```python
from build123d import *

# Parameters (mm, degrees)
F2_R = 12.599118
F3_R = 6.735102
F4_R = 3.026182
F5_R = 1.710135
F6_R = 1.408864


with BuildPart() as f1:
    # F0 (on Front) → F1 (revolve)
    with BuildSketch(Plane.XZ):
        Polygon((-9.7125, 0), (0, 0), (0, 22.078488), (-1.08705, 22.078488), (-3.406609, 20.364031), (-5.827018, 17.439371), (-6.936371, 12.598556), (-6.230419, 11.590051), (-7.944874, 11.18665), align=None)
    revolve(axis=Axis((0, 0, 11.039244), (0, 0, -1)))

    # F2
    f2_edges = [f1.edges().sort_by_distance(p)[0] for p in [
        (5.827018, 0, 17.439371),
    ]]
    fillet(f2_edges, radius=F2_R)

    # F3
    f3_edges = [f1.edges().sort_by_distance(p)[0] for p in [
        (3.406609, 0, 20.364031),
    ]]
    fillet(f3_edges, radius=F3_R)

    # F4
    f4_edges = [f1.edges().sort_by_distance(p)[0] for p in [
        (1.08705, 0, 22.078488),
    ]]
    fillet(f4_edges, radius=F4_R)

    # F5
    f5_edges = [f1.edges().sort_by_distance(p)[0] for p in [
        (7.944874, 0, 11.18665),
    ]]
    fillet(f5_edges, radius=F5_R)

    # F6
    f6_edges = [f1.edges().sort_by_distance(p)[0] for p in [
        (9.7125, 0, 0),
    ]]
    fillet(f6_edges, radius=F6_R)


solid = f1.part
```
For this review, take the finished solid that the model builds, in its own axes (mm). Round coordinates to 2 decimals unless told otherwise and drop trailing zeros. Loops run counter-clockwise (first coordinate to the right, second up) from the corner with the lowest first, then second, coordinate; pieces in that order, holes last.
(1) We need section A-A (z = 12). Give the boundary of the cut face in (x, y).
Returned:
outline: circle Ø13.03 at (0, 0)
(2) We need section B-B (z = 9.5). Give the boundary of the cut face in (x, y).
Returned:
outline: circle Ø16.42 at (0, 0)
(3) Wall thickness on line 1 along X through (y, z) = (1.25, 15.5); line 2 along Y through (x, z) = (-2.5, 12.25); line 3 along X through (y, z) = (8.5, 2.75): over which ranges is each line inside the solid? List them lowest first.
Returned:
line 1: x = -6.1 to 6.1
line 2: y = -6.21 to 6.21
line 3: x = -3.72 to 3.72
(4) Clearance check with flat-ended pins moving along their axes: P1, Ø6, axis at x = 6.5, y = 4.5, coming from the -Z side; P2, Ø4, axis at y = 4.5, z = 7, coming from the -X side; P3, Ø2, axis at x = -1.5, z = 19.5, coming from the +Y side; P4, Ø3, axis at y = 7, z = 14.5, coming from the -X side. State where each tip first meets the part, or that it passes through.
Returned:
P1: stops at z = 0
P2: stops at x = -8.32
P3: stops at y = 4.65
P4: stops at x = -3.55
